```python
from build123d import *

# Parameters (mm, degrees)
SKETCH1_R      = 2.6035
EXTRUDE1_DEPTH = 44.45


with BuildPart() as part:
    # Sketch1 → Extrude1 (new body)
    with BuildSketch(Plane.XY):
        with BuildLine():
            Line((813.038976674, 579.290424026), (813.038976674, 582.236824026))
            ThreePointArc((813.038976674, 582.236824026), (812.530976674, 582.744824026), (813.038976674, 583.252824026))
            Line((813.038976674, 583.252824026), (813.038976674, 584.484724026))
            ThreePointArc((813.038976674, 584.484724026), (811.934076674, 585.589624026), (810.829176674, 584.484724026))
            Line((810.829176674, 584.484724026), (810.829176674, 582.435874947))
            ThreePointArc((810.829176674, 582.435874947), (810.182743454, 581.495163196), (809.057340701, 581.685644565))
            Line((809.057340701, 581.685644565), (805.773323088, 584.969563516))
            ThreePointArc((805.773323088, 584.969563516), (805.085045004, 585.999619341), (804.843353394, 587.214661271))
            Line((804.843353394, 587.214661271), (804.843353394, 590.467068589))
            ThreePointArc((804.843353394, 590.467068589), (805.085043572, 591.682107061), (805.773317796, 592.712161052))
            Line((805.773317796, 592.712161052), (809.057121325, 595.995881407))
            ThreePointArc((809.057121325, 595.995881407), (810.18544278, 596.185153907), (810.829176674, 595.239352628))
            Line((810.829176674, 595.239352628), (810.829176674, 593.196924026))
            ThreePointArc((810.829176674, 593.196924026), (811.934076674, 592.092024026), (813.038976674, 593.196924026))
            Line((813.038976674, 593.196924026), (813.038976674, 594.428824026))
            ThreePointArc((813.038976674, 594.428824026), (812.530976674, 594.936824026), (813.038976674, 595.444824026))
            Line((813.038976674, 595.444824026), (813.038976674, 598.391224026))
            ThreePointArc((813.038976674, 598.391224026), (812.530976674, 598.899224026), (813.038976674, 599.407224026))
            Line((813.038976674, 599.407224026), (813.038976674, 599.432624026))
            ThreePointArc((813.038976674, 599.432624026), (812.42149919, 600.923346542), (810.930776674, 601.540824026))
            Line((810.930776674, 601.540824026), (810.905376674, 601.540824026))
            ThreePointArc((810.905376674, 601.540824026), (810.397376674, 601.032824026), (809.889376674, 601.540824026))
            Line((809.889376674, 601.540824026), (806.942976674, 601.540824026))
            ThreePointArc((806.942976674, 601.540824026), (806.434976674, 601.032824026), (805.926976674, 601.540824026))
            Line((805.926976674, 601.540824026), (804.695076674, 601.540824026))
            ThreePointArc((804.695076674, 601.540824026), (803.590176674, 600.435924026), (804.695076674, 599.331024026))
            Line((804.695076674, 599.331024026), (806.743925753, 599.331024026))
            ThreePointArc((806.743925753, 599.331024026), (807.684637504, 598.684590806), (807.494156135, 597.559188053))
            Line((807.494156135, 597.559188053), (804.210237184, 594.27517044))
            ThreePointArc((804.210237184, 594.27517044), (803.180181359, 593.586892356), (801.965139429, 593.345200745))
            Line((801.965139429, 593.345200745), (798.712732111, 593.345200745))
            ThreePointArc((798.712732111, 593.345200745), (797.497693639, 593.586890924), (796.467639648, 594.275165148))
            Line((796.467639648, 594.275165148), (793.183919293, 597.558968677))
            ThreePointArc((793.183919293, 597.558968677), (792.994646793, 598.687290132), (793.940448072, 599.331024026))
            Line((793.940448072, 599.331024026), (795.982876674, 599.331024026))
            ThreePointArc((795.982876674, 599.331024026), (797.087776674, 600.435924026), (795.982876674, 601.540824026))
            Line((795.982876674, 601.540824026), (794.750976674, 601.540824026))
            ThreePointArc((794.750976674, 601.540824026), (794.242976674, 601.032824026), (793.734976674, 601.540824026))
            Line((793.734976674, 601.540824026), (790.788576674, 601.540824026))
            ThreePointArc((790.788576674, 601.540824026), (790.280576674, 601.032824026), (789.772576674, 601.540824026))
            Line((789.772576674, 601.540824026), (789.747176674, 601.540824026))
            ThreePointArc((789.747176674, 601.540824026), (788.256454158, 600.923346542), (787.638976674, 599.432624026))
            Line((787.638976674, 599.432624026), (787.638976674, 599.407224026))
            ThreePointArc((787.638976674, 599.407224026), (788.146976674, 598.899224026), (787.638976674, 598.391224026))
            Line((787.638976674, 598.391224026), (787.638976674, 595.444824026))
            ThreePointArc((787.638976674, 595.444824026), (788.146976674, 594.936824026), (787.638976674, 594.428824026))
            Line((787.638976674, 594.428824026), (787.638976674, 593.196924026))
            ThreePointArc((787.638976674, 593.196924026), (788.743876674, 592.092024026), (789.848776674, 593.196924026))
            Line((789.848776674, 593.196924026), (789.848776674, 595.245773105))
            ThreePointArc((789.848776674, 595.245773105), (790.495209894, 596.186484856), (791.620612647, 595.996003487))
            Line((791.620612647, 595.996003487), (794.90463026, 592.712084536))
            ThreePointArc((794.90463026, 592.712084536), (795.592908344, 591.682028711), (795.834599954, 590.466986781))
            Line((795.834599954, 590.466986781), (795.834599954, 587.214579463))
            ThreePointArc((795.834599954, 587.214579463), (795.592909776, 585.999540991), (794.904635552, 584.969487))
            Line((794.904635552, 584.969487), (791.620832022, 581.685766645))
            ThreePointArc((791.620832022, 581.685766645), (790.492510568, 581.496494145), (789.848776674, 582.442295424))
            Line((789.848776674, 582.442295424), (789.848776674, 584.484724026))
            ThreePointArc((789.848776674, 584.484724026), (788.743876674, 585.589624026), (787.638976674, 584.484724026))
            Line((787.638976674, 584.484724026), (787.638976674, 583.252824026))
            ThreePointArc((787.638976674, 583.252824026), (788.146976674, 582.744824026), (787.638976674, 582.236824026))
            Line((787.638976674, 582.236824026), (787.638976674, 579.290424026))
            ThreePointArc((787.638976674, 579.290424026), (788.146976674, 578.782424026), (787.638976674, 578.274424026))
            Line((787.638976674, 578.274424026), (787.638976674, 578.249024026))
            ThreePointArc((787.638976674, 578.249024026), (788.256454158, 576.75830151), (789.747176674, 576.140824026))
            Line((789.747176674, 576.140824026), (789.772576674, 576.140824026))
            ThreePointArc((789.772576674, 576.140824026), (790.280576674, 576.648824026), (790.788576674, 576.140824026))
            Line((790.788576674, 576.140824026), (793.734976674, 576.140824026))
            ThreePointArc((793.734976674, 576.140824026), (794.242976674, 576.648824026), (794.750976674, 576.140824026))
            Line((794.750976674, 576.140824026), (795.982876674, 576.140824026))
            ThreePointArc((795.982876674, 576.140824026), (797.087776674, 577.245724026), (795.982876674, 578.350624026))
            Line((795.982876674, 578.350624026), (793.934027595, 578.350624026))
            ThreePointArc((793.934027595, 578.350624026), (792.993315844, 578.997057246), (793.183797213, 580.122459999))
            Line((793.183797213, 580.122459999), (796.467716164, 583.406477612))
            ThreePointArc((796.467716164, 583.406477612), (797.497771989, 584.094755696), (798.712813919, 584.336447306))
            Line((798.712813919, 584.336447306), (801.965221237, 584.336447306))
            ThreePointArc((801.965221237, 584.336447306), (803.180259709, 584.094757128), (804.2103137, 583.406482904))
            Line((804.2103137, 583.406482904), (807.494034055, 580.122679374))
            ThreePointArc((807.494034055, 580.122679374), (807.683306555, 578.99435792), (806.737505276, 578.350624026))
            Line((806.737505276, 578.350624026), (804.695076674, 578.350624026))
            ThreePointArc((804.695076674, 578.350624026), (803.590176674, 577.245724026), (804.695076674, 576.140824026))
            Line((804.695076674, 576.140824026), (805.926976674, 576.140824026))
            ThreePointArc((805.926976674, 576.140824026), (806.434976674, 576.648824026), (806.942976674, 576.140824026))
            Line((806.942976674, 576.140824026), (809.889376674, 576.140824026))
            ThreePointArc((809.889376674, 576.140824026), (810.397376674, 576.648824026), (810.905376674, 576.140824026))
            Line((810.905376674, 576.140824026), (810.930776674, 576.140824026))
            ThreePointArc((810.930776674, 576.140824026), (812.42149919, 576.75830151), (813.038976674, 578.249024026))
            Line((813.038976674, 578.249024026), (813.038976674, 578.274424026))
            ThreePointArc((813.038976674, 578.274424026), (812.530976674, 578.782424026), (813.038976674, 579.290424026))
        make_face()
        with Locations((800.338976674, 588.840824026)):
            Circle(SKETCH1_R, mode=Mode.SUBTRACT)
    extrude(amount=-EXTRUDE1_DEPTH)


solid = part.part
```
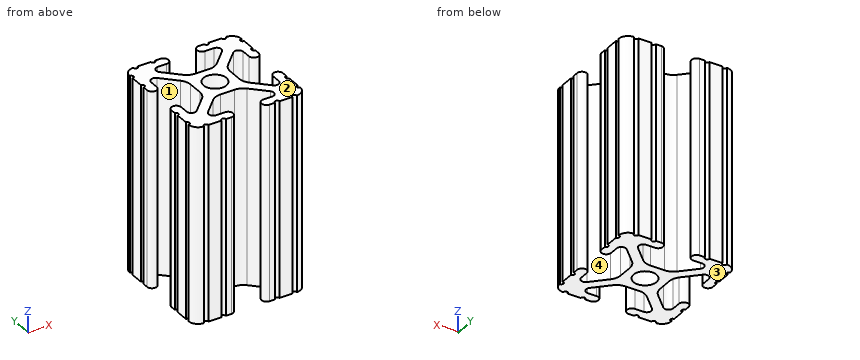
The model under review builds one solid part; all positions refer to its coordinate system, in mm. Face numbers are marked on the shaded views. A direction names the side the tool comes from. Round coordinates to 2 decimals unless told otherwise and drop trailing zeros. Loops run counter-clockwise (first coordinate to the right, second up) from the corner with the lowest first, then second, coordinate; pieces in that order, holes last. Notation, with made-up numbers: M 12,24 L 70,24 A21 ccw 70,36 Z; hole C 3.25,-0.75 d8. An arc over 180 degrees is marked long. Answer as a JSON object with one key per item and string values.
(1) Take a section at B-B on y = 600. Give the boundary of the cut face in (x, z), and give its area (3 significant figures).
Resolved:
{"outline": "M 787.72,-44.45 L 797,-44.45 L 797,0 L 787.72,0 Z; M 803.68,-44.45 L 812.96,-44.45 L 812.96,0 L 803.68,0 Z", "area": "825 mm²"}
(2) Take a section at A-A on x = 800. Give the boundary of the cut face in (y, z), and give its area (3 significant figures).
Resolved:
{"outline": "M 584.34,-44.45 L 586.26,-44.45 L 586.26,0 L 584.34,0 Z; M 591.42,-44.45 L 593.35,-44.45 L 593.35,0 L 591.42,0 Z", "area": "171 mm²"}
(3) Draft analysis for pull direction X (two halves, no side actions). For the marked faces 1 and 2, state which applies: released by +X, released by -X, zero draft, split by the parting line, or undercut.
Resolved:
{"face 1": "undercut", "face 2": "zero draft"}
(4) Tool access review of the marked faces 3 and 4: name each direction out of +Z, -Z, +X, -X, +Y, -Y from which nothing blocks a thin tool from reaching the whole face with its end or side.
Resolved:
{"face 3": "-Z, +X, -X, +Y, -Y", "face 4": "+Z, -Z"}
(5) Clearance check with flat-ended pins moving along their axes: P1, Ø1.6, axis at x = 800.5, z = -31, coming from the +Y side; P2, Ø1.6, axis at x = 800.5, z = -24, coming from the -Y side; P3, Ø1.6, axis at y = 588.5, z = -19.5, coming from the +X side; P4, Ø3, axis at x = 800.34, y = 588.84, coming from the +Z side. State where each tip first meets the part, or that it passes through.
Resolved:
{"P1": "y = 593.35", "P2": "y = 584.34", "P3": "x = 804.84", "P4": "through"}
(6) To check wall thickness, follow line 1 along X through (y, z) = (589, -2); line 2 along Y through (x, z) = (805.25, -13.5); line 3 along X through (y, z) = (581.75, -8). State the ranges of each line that lie inside material, in increasing order.
Resolved:
{"line 1": "795.83 to 797.74, 802.94 to 804.84", "line 2": "576.14 to 578.35, 582.37 to 585.66, 592.02 to 595.31, 599.33 to 601.54", "line 3": "787.64 to 790.13, 791.69 to 794.81, 805.87 to 808.99, 810.55 to 813.04"}
